```python
from build123d import *

# Parameters (mm, degrees)
F1_DEPTH = 0.5
F2_R     = 1.1
F3_DEPTH = 0.501


with BuildPart() as f1:
    # F0 (on Front) → F1 (new body)
    with BuildSketch(Plane.XZ):
        Polygon((39.504941, 126.711226), (-196.495059, 126.711226), (-196.495059, 401.711226), (-260.495059, 401.711226), (-260.495059, 126.711226), (-260.495059, -473.288774), (39.504941, -473.288774), align=None)
    extrude(amount=F1_DEPTH)

    # F2 (on face) → F3 (cut, through all)
    with BuildSketch(Plane.XZ.offset(0.5)):
        with Locations((-255.495059, 386.711226)):
            Circle(F2_R)
        with Locations((-201.495059, 386.711226)):
            Circle(F2_R)
    extrude(amount=-F3_DEPTH, mode=Mode.SUBTRACT)


solid = f1.part
```
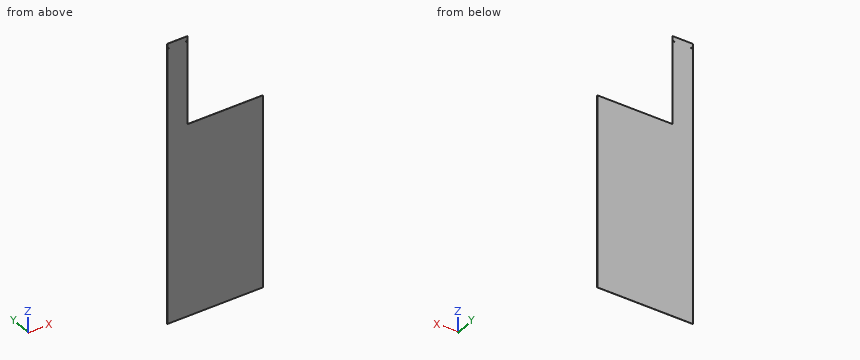
Geometry check sheet. Reference: the model listing, model coordinates, mm. Coordinates: 2 decimals unless noted, no trailing zeros. Write each loop counter-clockwise with the first axis right and the second up, starting at its lowest first coordinate (ties: lowest second). Pieces come first, ordered by that corner, then holes. Notation, with made-up numbers: M 83,31 L 129,31 A23 ccw 129,58 Z; hole C 7.5,-37 d4. An arc over 180 degrees is marked long. One line per item, written item: value. Start each with the question number.
(1) Sectioned sample at C-C, the plane z = 181. Enter the section's corners in (x, y), and give its area (3 significant figures).
(2) Sectioned sample at A-A, the plane y = -0.4. Enter the section's corners in (x, z).
(3) Scan lines: line 1 along Z through (x, y) = (-22, -0.3); line 2 along X through (y, z) = (-0.05, 286). Record each from-to range of solid material in increasing order. Write a range as [from, to].
(4) Depth check by flat-ended pin: pin 1 (1.8 mm diameter, centred on x = -255.5, z = 386.71, fed in from +Y). Enter the tip coordinate at first touch or a pass-through.
(5) Sectioned sample at B-B, the plane x = -132. Enter the section's corners in (y, z), and give its area (3 significant figures).
Filled sheet:
1. outline: M -260.5,-0.5 L -196.5,-0.5 L -196.5,0 L -260.5,0 Z
1. area: 32.0 mm²
2. outline: M -260.5,-473.29 L 39.5,-473.29 L 39.5,126.71 L -196.5,126.71 L -196.5,401.71 L -260.5,401.71 Z; hole C -255.5,386.71 d2.2; hole C -201.5,386.71 d2.2
3. line 1: [-473.29, 126.71]
3. line 2: [-260.5, -196.5]
4. pin 1: through
5. outline: M -0.5,-473.29 L 0,-473.29 L 0,126.71 L -0.5,126.71 Z
5. area: 300 mm²
